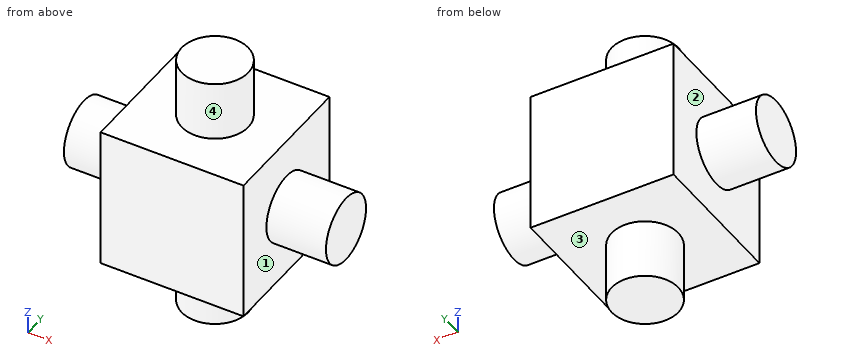
from build123d import *

# Parameters (mm, degrees)
SKETCH_1_W      = 6
SKETCH_1_H      = 6
EXTRUDE_1_DEPTH = 6
SKETCH_2_R      = 1.4
EXTRUDE_2_DEPTH = 5.5
SKETCH_3_R      = 1.4
EXTRUDE_3_DEPTH = 5.5


with BuildPart() as part:
    # 草图1 → 凸台-拉伸1 (new body)
    with BuildSketch(Plane(origin=(0, 0, 0), x_dir=(1, 0, 0), z_dir=(0, 1, 0))):
        Rectangle(SKETCH_1_W, SKETCH_1_H)
    extrude(amount=EXTRUDE_1_DEPTH)

    # 草图2 → 凸台-拉伸2 (add, symmetric)
    with BuildSketch(Plane.XY):
        with Locations((0, 3)):
            Circle(SKETCH_2_R)
    extrude(amount=EXTRUDE_2_DEPTH, both=True)

    # 草图3 → 凸台-拉伸3 (add, symmetric)
    with BuildSketch(Plane(origin=(0, 0, 0), x_dir=(0, 0, -1), z_dir=(1, 0, 0))):
        with Locations((0, 3)):
            Circle(SKETCH_3_R)
    extrude(amount=EXTRUDE_3_DEPTH, both=True)


solid = part.part
Geometry check sheet. Reference: the model listing, model coordinates, mm. Face numbers are marked on the shaded views. A direction names the side the tool comes from. Give positions to 0.01 mm unless a question says otherwise; leave off trailing zeros. Loops run counter-clockwise (first coordinate to the right, second up) from the corner with the lowest first, then second, coordinate; pieces in that order, holes last. Notation, with made-up numbers: (64.25, -17) -> (115.25, -17) arc R25 cw to (115.25, 14) -> close; hole circle Ø5 at (72, -33). An arc over 180 degrees is marked (long way). Answer in a Markdown table with one row per item. Add a question column.
1) Cross-section at B-B on x = 0. Record the boundary of the cut face in (y, z), and give its area (3 significant figures).
2) Material ranges on probe 1 along Z at (x, y) = (1.5, 2.1); probe 2 along Y at (x, z) = (3.5, 0), recorded low to high. Write a range as from..to.
3) Cross-section at C-C on z = 0. Record the boundary of the cut face in (x, y), and give its area (3 significant figures).
4) Cross-section at A-A on y = 3. Record the boundary of the cut face in (x, z), and give its area (3 significant figures).
5) Gauge pin test, flat end, axial feed: P1, Ø1.5, axis at x = 2.5, z = -2, coming from the -Y side. Record the tip position at first contact, or that the pin passes through.
6) Cross-section at D-D on y = 1.9. Record the boundary of the cut face in (x, z), and give its area (3 significant figures).
7) Set-up check for the marked faces 1, 2, 3 and 4: record each of +Z, -Z, +X, -X, +Y, -Y from which the full face is reachable in a straight line by a thin tool's end or side.
Outcome:
| question | item | result |
|---|---|---|
| 1 | outline | (0, -3) -> (1.6, -3) -> (1.6, -5.5) -> (4.4, -5.5) -> (4.4, -3) -> (6, -3) -> (6, 3) -> (4.4, 3) -> (4.4, 5.5) -> (1.6, 5.5) -> (1.6, 3) -> (0, 3) -> close |
| 1 | area | 50.0 mm^2 |
| 2 | probe 1 | z = -3..3 |
| 2 | probe 2 | y = 1.6..4.4 |
| 3 | outline | (-5.5, 1.6) -> (-3, 1.6) -> (-3, 0) -> (3, 0) -> (3, 1.6) -> (5.5, 1.6) -> (5.5, 4.4) -> (3, 4.4) -> (3, 6) -> (-3, 6) -> (-3, 4.4) -> (-5.5, 4.4) -> close |
| 3 | area | 50.0 mm^2 |
| 4 | outline | (-5.5, -1.4) -> (-3, -1.4) -> (-3, -3) -> (-1.4, -3) -> (-1.4, -5.5) -> (1.4, -5.5) -> (1.4, -3) -> (3, -3) -> (3, -1.4) -> (5.5, -1.4) -> (5.5, 1.4) -> (3, 1.4) -> (3, 3) -> (1.4, 3) -> (1.4, 5.5) -> (-1.4, 5.5) -> (-1.4, 3) -> (-3, 3) -> (-3, 1.4) -> (-5.5, 1.4) -> close |
| 4 | area | 64.0 mm^2 |
| 5 | P1 | stops at y = 0 |
| 6 | outline | (-5.5, -0.87) -> (-3, -0.87) -> (-3, -3) -> (-0.87, -3) -> (-0.87, -5.5) -> (0.87, -5.5) -> (0.87, -3) -> (3, -3) -> (3, -0.87) -> (5.5, -0.87) -> (5.5, 0.87) -> (3, 0.87) -> (3, 3) -> (0.87, 3) -> (0.87, 5.5) -> (-0.87, 5.5) -> (-0.87, 3) -> (-3, 3) -> (-3, 0.87) -> (-5.5, 0.87) -> close |
| 6 | area | 53.3 mm^2 |
| 7 | face 1 | +X |
| 7 | face 2 | -X |
| 7 | face 3 | -Z |
| 7 | face 4 | +Z |
